from build123d import *

# Parameters (mm, degrees)
SKETCH1_W           = 12.5
SKETCH1_H           = 15
BOSS_EXTRUDE1_DEPTH = 2
SKETCH4_W           = 4
SKETCH4_H           = 15
BOSS_EXTRUDE2_DEPTH = 12
BOSS_EXTRUDE3_DEPTH = 4
SKETCH5_R           = 3.5
CUT_EXTRUDE2_DEPTH  = 19.013883535
SKETCH9_R           = 5.9
CUT_EXTRUDE4_DEPTH  = 3
BOSS_EXTRUDE4_DEPTH = 2


with BuildPart() as part:
    # Sketch1 → Boss-Extrude1 (new body)
    with BuildSketch(Plane(origin=(0, 0, 0), x_dir=(1, 0, 0), z_dir=(0, 1, 0))):
        Rectangle(SKETCH1_W, SKETCH1_H)
    extrude(amount=BOSS_EXTRUDE1_DEPTH)

    # Sketch4 → Boss-Extrude2 (add)
    with BuildSketch(Plane(origin=(0, 2, 0), x_dir=(1, 0, 0), z_dir=(0, 1, 0))):
        with Locations((4.25, 0)):
            Rectangle(SKETCH4_W, SKETCH4_H)
    extrude(amount=BOSS_EXTRUDE2_DEPTH)

    # Sketch8 → Boss-Extrude3 (add)
    with BuildSketch(Plane.XY.offset(7.5)):
        Polygon((2.25, 2), (2.25, 7), (-0.25, 2), align=None)
    boss_extrude3 = extrude(amount=-BOSS_EXTRUDE3_DEPTH)

    # Sketch5 → Cut-Extrude2 (cut, through all)
    with BuildSketch(Plane.ZY.offset(-2.25)):
        with Locations((0, 7.965)):
            Circle(SKETCH5_R)
    extrude(amount=-CUT_EXTRUDE2_DEPTH, mode=Mode.SUBTRACT)

    # Sketch10 → CSK for #6 Flat Head Machine Screw (100)1 (revolve, cut)
    with BuildSketch(Plane(origin=(-2.25, 2, 0), x_dir=(0, 0, 1), z_dir=(1, 0, 0))):
        Polygon((0, 0), (0, 2), (2.15265, 2), (2.15265, 1.166893902), (3.5433, 0), align=None)
    revolve(axis=Axis((-2.25, 8.35, 0), (0, -1, 0)), mode=Mode.SUBTRACT)

    # Mirror1: Boss-Extrude3 across plane
    add(boss_extrude3.mirror(Plane.XY))

    # Sketch9 → Cut-Extrude4 (cut)
    with BuildSketch(Plane.ZY.offset(-2.25)):
        with Locations((0, 7.965)):
            Circle(SKETCH9_R)
    extrude(amount=CUT_EXTRUDE4_DEPTH, mode=Mode.SUBTRACT)

    # Sketch12 → Boss-Extrude4 (add)
    with BuildSketch(Plane.XY.offset(7.5)):
        Polygon((2.25, 14), (-6.25, 2), (-6.25, 0), (6.25, 0), (6.25, 14), align=None)
    boss_extrude4 = extrude(amount=BOSS_EXTRUDE4_DEPTH)

    # Mirror2: Boss-Extrude4 across plane
    add(boss_extrude4.mirror(Plane.XY))


solid = part.part
Geometry check sheet. Reference: the model listing, model coordinates, mm. A direction names the side the tool comes from. Round coordinates to 2 decimals unless told otherwise and drop trailing zeros. Write each loop counter-clockwise with the first axis right and the second up, starting at its lowest first coordinate (ties: lowest second). Pieces come first, ordered by that corner, then holes. Notation, with made-up numbers: (50.25, -34) - (94.25, -34) arc R22 cw to (94.25, -24) - close; hole circle Ø9 at (84.25, 12). An arc over 180 degrees is marked (long way). One line per item, written item: value.
1. Depth check by flat-ended pin: pin 1 Ø3.5 at (x, z) = (-2.25, 0) entering from -Y; pin 2 Ø2 at (y, z) = (10, -6) entering from -X; pin 3 Ø7 at (x, z) = (-3.5, -3) entering from +Y; pin 4 Ø4 at (y, z) = (5, -5) entering from -X. Enter the tip coordinate at first touch or a pass-through.
The answers:
pin 1: passes through
pin 2: stops at x = 2.25
pin 3: stops at y = 2.43
pin 4: stops at x = 0.25
2. Cross-section at D-D on z = 6.5. Record the boundary of the cut face in (x, y).
The answers:
outline: (-6.25, 0) - (6.25, 0) - (6.25, 14) - (2.25, 14) - (2.25, 7) - (-0.25, 2) - (-6.25, 2) - close
3. Cross-section at C-C on x = -2.25. Record the boundary of the cut face in (y, z).
The answers:
outline: (0, -9.5) - (7.65, -9.5) - (7.65, -7.5) - (2, -7.5) - (2, -3.54) - (0.83, -2.15) - (0, -2.15) - close; (0, 2.15) - (0.83, 2.15) - (2, 3.54) - (2, 7.5) - (7.65, 7.5) - (7.65, 9.5) - (0, 9.5) - close
4. Cross-section at B-B on y = 6.75. Record the boundary of the cut face in (x, z) (3 decimals).
The answers:
outline: (-2.885, -9.5) - (6.25, -9.5) - (6.25, -3.282) - (2.25, -3.282) - (2.25, -5.774) - (2.125, -5.774) - (2.125, -7.5) - (-2.885, -7.5) - close; (-2.885, 7.5) - (2.125, 7.5) - (2.125, 5.774) - (2.25, 5.774) - (2.25, 3.282) - (6.25, 3.282) - (6.25, 9.5) - (-2.885, 9.5) - close
5. Set-up check for faces 1 (the face through (0.74, 3.98, 5.97)), 2 (the face through (4, 14, 0)): record each of +Z, -Z, +X, -X, +Y, -Y from which the full face is reachable in a straight line by a thin tool's end or side.
The answers:
face 1: -X, +Y
face 2: +Z, -Z, +X, -X, +Y
6. Cross-section at A-A on z = 0. Record the boundary of the cut face in (x, y) (3 decimals).
The answers:
outline: (-6.25, 0) - (-4.403, 0) - (-4.403, 0.833) - (-5.793, 2) - (-6.25, 2) - close; (-0.097, 0) - (6.25, 0) - (6.25, 4.465) - (2.25, 4.465) - (2.25, 2) - (1.293, 2) - (-0.097, 0.833) - close; (2.25, 11.465) - (6.25, 11.465) - (6.25, 14) - (2.25, 14) - close
7. Scan lines: L1, parallel to Z at x = -2.25, y = 0.5; L2, parallel to X at y = 0.3, z = 0; L3, parallel to Z at x = 1.25, y = 2.5. Record each from-to range of solid material in increasing order.
The answers:
L1: z = -9.5 to -2.15, 2.15 to 9.5
L2: x = -6.25 to -4.4, -0.1 to 6.25
L3: z = -9.5 to -3.5, 3.5 to 9.5
